Here's the drawing with two shaded views (mm, measured from the low corner). I have some questions. A direction names the side the tool comes from. Round coordinates to 2 decimals unless told otherwise and drop trailing zeros. Write each loop counter-clockwise with the first axis right and the second up, starting at its lowest first coordinate (ties: lowest second). Pieces come first, ordered by that corner, then holes. Notation, with made-up numbers: M -7,34 L 20,34 A22 ccw 20,60 Z; hole C -18.75,-38.75 d7. An arc over 180 degrees is marked long. Use one line per item in the form item = value. Start each with the question number.
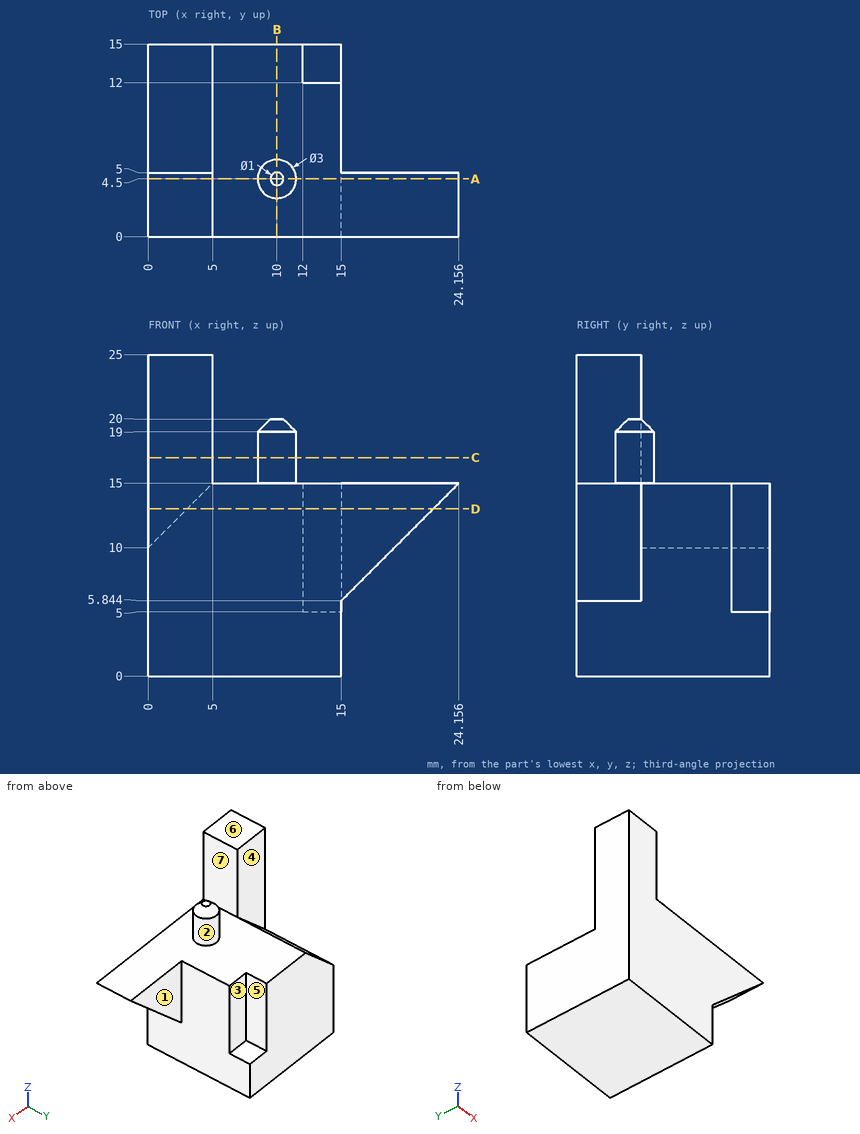
1. If we section it at A-A (y = 4.5): List the corners of the cut face in (x, z) for me, and give its area (3 significant figures).
2. Which directions (+Z, -Z, +X, -X, +Y, -Y) give clear straight access to the entire face, cutting with the end or side of a thin tool? Please do the marked faces 1, 2, 3 and 4.
3. Please list where these lines run through material, in increasing order: line 1 along X through (y, z) = (7.5, 6.5); line 2 along Z through (x, y) = (1.5, 7).
4. If we mould it in two halves opening along X, with no side actions, what happens to the marked faces 5, 6 and 7? For each: pulls with the +X half, pulls with the -X half, needs draft (parallel to the pull), parting line crosses it, or undercut.
5. If we section it at B-B (x = 10): List the corners of the cut face in (y, z) for me, and give its area (3 significant figures).
6. If we section it at C-C (z = 17): List the corners of the cut face in (x, y) for me.
7. If we section it at D-D (z = 13): List the corners of the cut face in (x, y) for me, and give its area (3 significant figures).
8. Will these pins go through, and if not, where does the flat tip stop? pin 1 (10 mm diameter, centred on x = 19, z = 16.5, fed in from +Y); pin 2 (1.5 mm diameter, centred on x = 3.5, z = 17.5, fed in from +Y); pin 3 (2.5 mm diameter, centred on x = 13.5, y = 14, fed in from +Z).
Model answer:
q1.outline = M 0,0 L 15,0 L 15,5.84 L 24.16,15 L 11.5,15 L 11.5,19 L 10.5,20 L 9.5,20 L 8.5,19 L 8.5,15 L 5,15 L 5,25 L 0,25 Z
q1.area = 331 mm2
q2.face_1 = +Z, -Z, +X, +Y
q2.face_2 = +Z
q2.face_3 = +Z, +X, +Y
q2.face_4 = +Z, -X, +Y
q3.line_1 = 0 to 15
q3.line_2 = 0 to 11.5
q4.face_5 = pulls with the +X half
q4.face_6 = needs draft
q4.face_7 = undercut
q5.outline = M 0,0 L 15,0 L 15,15 L 6,15 L 6,19 L 5,20 L 4,20 L 3,19 L 3,15 L 0,15 Z
q5.area = 239 mm2
q6.outline = M 0,0 L 5,0 L 5,5 L 0,5 Z; C 10,4.5 d3
q7.outline = M 0,0 L 22.16,0 L 22.16,5 L 15,5 L 15,12 L 12,12 L 12,15 L 3,15 L 3,5 L 0,5 Z
q7.area = 222 mm2
q8.pin_1 = 12
q8.pin_2 = 5
q8.pin_3 = 5
